from build123d import *

# Parameters (mm, degrees)
F1_DEPTH = 3.5
F2_T     = -0.5
F4_D     = 5.5


with BuildPart() as f1:
    # F0 (on Front) → F1 (new body, symmetric)
    with BuildSketch(Plane.XZ):
        Polygon((-5.5, 13), (-7.5, 0), (7.5, 0), (5.5, 13), align=None)
    extrude(amount=F1_DEPTH, both=True)

    # F2
    f2_openings = [f1.faces().sort_by_distance(p)[0] for p in [
        (0, 0, 0),
    ]]
    offset(amount=F2_T, openings=f2_openings)

    # F4 (through all)
    with Locations(Plane(origin=(7.3265895954, 0, 1.1271676301), x_dir=(0, 1, 0), z_dir=(0.9883716977, 0, 0.1520571843))):
        with Locations((0, 8.0125175561)):
            Hole(F4_D / 2)


solid = f1.part
The listing builds one solid part. Answer for the finished solid, in the listing's coordinates (mm). A direction names the side the tool comes from. Give positions to 0.01 mm unless a question says otherwise; leave off trailing zeros. Write each loop counter-clockwise with the first axis right and the second up, starting at its lowest first coordinate (ties: lowest second). Pieces come first, ordered by that corner, then holes.
Item 1: Determine the mould class of faces 3 (the flat face through (0, 3, 6)), 4 (the flat face through (6.736, -0.049, 4.965)), 5 (the flat face through (0, 0, 13)) for opening direction X: released by +X, released by -X, zero draft, split by the parting line, or undercut.
Item 2: Section A-A, the plane y = 1 is taken. Write down the section's boundary in (x, z).
Item 3: Section D-D, the plane y = -2 is taken. Write down the section's boundary in (x, z).
Item 4: Flat-ended cylindrical pins translate along their axes: P1, Ø3, axis at x = -3.5, y = -1, coming from the -Z side; P2, Ø3, axis at y = 2.5, z = 4.5, coming from the +X side. Find the tip coordinate at first contact, or state that the pin passes through.
Item 5: Section B-B, the plane x = -3.5 is taken. Write down the section's boundary in (y, z), plus the area to 3 significant figures.
Item 6: Which of the six approach directions +Z, -Z, +X, -X, +Y, -Y give full straight-line access (tool end or side, diameter ignored) to faces 1 (the flat face through (0, 3.5, 7)), 2 (the flat face through (-6.233, -2.042, 4.949))?
Item 7: Find the intervals of material crossed by line 1 along Y through (x, z) = (1, 7); line 2 along Z through (x, y) = (0.5, 0); line 3 along X through (y, z) = (-2, 3.5), in increasing order.
Item 8: Section C-C, the plane z = 3.5 is taken. Write down the section's boundary in (x, y).
Completed:
1. face 3: undercut
1. face 4: released by +X
1. face 5: zero draft
2. outline: (-7.5, 0) - (-6.99, 0) - (-6.29, 4.55) - (-6.81, 4.47) - close; (-6, 9.78) - (-5.48, 9.86) - (-5.07, 12.5) - (5.07, 12.5) - (5.22, 11.5) - (5.72, 11.58) - (5.5, 13) - (-5.5, 13) - close; (6, 6.44) - (6.99, 0) - (7.5, 0) - (6.5, 6.51) - close
3. outline: (-7.5, 0) - (-6.99, 0) - (-6.19, 5.25) - (-6.71, 5.17) - close; (-6.1, 9.08) - (-5.59, 9.16) - (-5.07, 12.5) - (5.07, 12.5) - (5.33, 10.84) - (5.82, 10.91) - (5.5, 13) - (-5.5, 13) - close; (5.9, 7.1) - (6.99, 0) - (7.5, 0) - (6.4, 7.18) - close
4. P1: stops at z = 12.5
4. P2: stops at x = 7.04
5. outline: (-3.5, 0) - (-3, 0) - (-3, 12.5) - (3, 12.5) - (3, 0) - (3.5, 0) - (3.5, 13) - (-3.5, 13) - close
5. area: 16.0 mm2
6. face 1: +Z, -Z, +X, -X, +Y
6. face 2: -Z
7. line 1: y = -3.5 to -3, 3 to 3.5
7. line 2: z = 12.5 to 13
7. line 3: x = -6.96 to -6.46, 6.46 to 6.96
8. outline: (-6.96, -3.5) - (6.96, -3.5) - (6.96, 3.5) - (-6.96, 3.5) - close; hole (-6.46, -3) - (6.46, -3) - (6.46, 3) - (-6.46, 3) - close
